```python
from build123d import *

# Parameters (mm, degrees)
ESBO_O1_R                = 1.5
ESBO_O1_W                = 5
ESBO_O1_H                = 35
RESSALTO_EXTRUS_O1_DEPTH = 3
ESBO_O2_W                = 25
ESBO_O2_H                = 5
RESSALTO_EXTRUS_O2_DEPTH = 15
FILETE5_R                = 5
FILETE6_R                = 5
FILETE7_R                = 5
FILETE8_R                = 5
ESBO_O3_R                = 1
ESBO_O3_W                = 4
ESBO_O3_H                = 4
CORTE_EXTRUS_O1_DEPTH    = 5
CORTE_EXTRUS_O2_START    = -5
ESBO_O4_R                = 1
ESBO_O4_W                = 4
ESBO_O4_H                = 4
CORTE_EXTRUS_O2_DEPTH    = 5


with BuildPart() as part:
    # Esboço1 → Ressalto-extrusão1 (new body)
    with BuildSketch(Plane.XY):
        Polygon((-24.430369357, 7.066666667), (10.569630643, 7.066666667), (10.569630643, 2.066666667), (5.569630643, 2.066666667), (5.569630643, -32.933333333), (10.569630643, -32.933333333), (10.569630643, -37.933333333), (-24.430369357, -37.933333333), (-24.430369357, -32.933333333), (-19.430369357, -32.933333333), (-19.430369357, 2.066666667), (-24.430369357, 2.066666667), align=None)
        with Locations((-14.430369357, -4.933333333)):
            Circle(ESBO_O1_R, mode=Mode.SUBTRACT)
        with Locations((-14.430369357, -11.933333333)):
            Circle(ESBO_O1_R, mode=Mode.SUBTRACT)
        with Locations((-14.430369357, -18.933333333)):
            Circle(ESBO_O1_R, mode=Mode.SUBTRACT)
        with Locations((0.569630643, -4.933333333)):
            Circle(ESBO_O1_R, mode=Mode.SUBTRACT)
        with Locations((0.569630643, -18.933333333)):
            Circle(ESBO_O1_R, mode=Mode.SUBTRACT)
        with Locations((0.569630643, -25.933333333)):
            Circle(ESBO_O1_R, mode=Mode.SUBTRACT)
        with Locations((-14.430369357, -25.933333333)):
            Circle(ESBO_O1_R, mode=Mode.SUBTRACT)
        with Locations((0.569630643, -11.933333333)):
            Circle(ESBO_O1_R, mode=Mode.SUBTRACT)
        with Locations((-21.930369357, 4.566666667)):
            Circle(ESBO_O1_R, mode=Mode.SUBTRACT)
        with Locations((8.069630643, 4.566666667)):
            Circle(ESBO_O1_R, mode=Mode.SUBTRACT)
        with Locations((-21.930369357, -35.433333333)):
            Circle(ESBO_O1_R, mode=Mode.SUBTRACT)
        with Locations((8.069630643, -35.433333333)):
            Circle(ESBO_O1_R, mode=Mode.SUBTRACT)
        with Locations((-6.930369357, -15.433333333)):
            Rectangle(ESBO_O1_W, ESBO_O1_H, mode=Mode.SUBTRACT)
    extrude(amount=-RESSALTO_EXTRUS_O1_DEPTH)

    # Esboço2 → Ressalto-extrusão2 (add)
    with BuildSketch(Plane.XY):
        with Locations((-6.930369357, 4.566666667)):
            Rectangle(ESBO_O2_W, ESBO_O2_H)
        with Locations((-6.930369357, -35.433333333)):
            Rectangle(ESBO_O2_W, ESBO_O2_H)
    extrude(amount=RESSALTO_EXTRUS_O2_DEPTH)

    # Filete5
    filete5_edges = [part.edges().sort_by_distance(p)[0] for p in [
        (5.569630643, -35.433333333, 15),
    ]]
    fillet(filete5_edges, radius=FILETE5_R)

    # Filete6
    filete6_edges = [part.edges().sort_by_distance(p)[0] for p in [
        (-19.430369357, -35.433333333, 15),
    ]]
    fillet(filete6_edges, radius=FILETE6_R)

    # Filete7
    filete7_edges = [part.edges().sort_by_distance(p)[0] for p in [
        (-19.430369357, 4.566666667, 15),
    ]]
    fillet(filete7_edges, radius=FILETE7_R)

    # Filete8
    filete8_edges = [part.edges().sort_by_distance(p)[0] for p in [
        (5.569630643, 4.566666667, 15),
    ]]
    fillet(filete8_edges, radius=FILETE8_R)

    # Esboço3 → Corte-extrusão1 (cut)
    with BuildSketch(Plane(origin=(0, -37.933333333, 0), x_dir=(-1, 0, 0), z_dir=(0, -1, 0))):
        with Locations(Location((13.180369357, -6, 0), (0, 0, 180))):
            Circle(ESBO_O3_R)
        with Locations(Location((0.680369357, -6.000000354, 0), (0, 0, 180))):
            Circle(ESBO_O3_R)
        with Locations((6.930369357, -6)):
            Rectangle(ESBO_O3_W, ESBO_O3_H)
    extrude(amount=-CORTE_EXTRUS_O1_DEPTH, mode=Mode.SUBTRACT)

    # Esboço4 → Corte-extrusão2 (cut)
    with BuildSketch(Plane(origin=(0, 7.066666667, 0), x_dir=(1, 0, 0), z_dir=(0, 1, 0)).offset(CORTE_EXTRUS_O2_START)):
        with Locations((-13.180369357, -6)):
            Circle(ESBO_O4_R)
        with Locations(Location((-0.680369357, -6, 0), (0, 0, 359.999979706))):
            Circle(ESBO_O4_R)
        with Locations((-6.930369357, -6)):
            Rectangle(ESBO_O4_W, ESBO_O4_H)
    extrude(amount=CORTE_EXTRUS_O2_DEPTH, mode=Mode.SUBTRACT)


solid = part.part
```
The listing builds one solid part. Answer for the finished solid, in the listing's coordinates (mm). A direction names the side the tool comes from. Give positions to 0.01 mm unless a question says otherwise; leave off trailing zeros. Loops run counter-clockwise (first coordinate to the right, second up) from the corner with the lowest first, then second, coordinate; pieces in that order, holes last. Notation, with made-up numbers: (-37, 6.5) - (-33, 6.5) arc R22 ccw to (-33, 28.5) - close; hole circle Ø2 at (60, 59). An arc over 180 degrees is marked (long way). Answer as CSV lines item,"result". Start each with the question number.
Item 1: For faces 1 (the face through (-23, 6, 0)), 2 (the face through (5.57, -35, 5)), 3 (the face through (8, 2.067, -1)), 4 (the face through (-4.93, 5, 6)), 5 (the face through (-19.43, -16, -1)), determine the directions among +Z, -Z, +X, -X, +Y, -Y from which every point of the face is accessible in a straight line to the end or side of a thin tool.
Item 2: A cutting plane is placed at C-C on z = 6. Count the separate pieces of the cut face and the enclosed holes in it, then the cut area to 3 significant figures.
Item 3: A cutting plane is placed at A-A on z = 3.25. Determine the outline of the cut face in (x, y), then the cut area to 3 significant figures.
Item 4: The mould has two halves that part along X. Classify faces 6 (the face through (-7, 7.067, 2)), 7 (the face through (-0.81, 4.53, 5.01)), 8 (the face through (-17.9, -35.4, 13.6)), 9 (the face through (10.57, 5, -1)): +X half, -X half, draft (parallel to the pull), parting line (faces both ways), or undercut.
Item 5: Find the intervals of material crossed by line 1 (X direction, y = -3, z = -0.5); line 2 (Y direction, x = -12.5, z = 9.5); line 3 (Y direction, x = -15, z = -0.25), in increasing order. Write a range as from..to.
Item 6: A cutting plane is placed at D-D on y = -28.5. Determine the outline of the cut face in (x, z).
Item 7: A cutting plane is placed at B-B on x = -8. Determine the outline of the cut face in (y, z), then the cut area to 3 significant figures.
Item 8: Each of these flat-tipped pins is pushed along its axis until it touches: pin 1 (4 mm diameter, centred on y = 4, z = 6.5, fed in from -X); pin 2 (12 mm diameter, centred on x = -17, y = -10.5, fed in from +Z); pin 3 (8 mm diameter, centred on y = -21, z = 0, fed in from +X). Where does it stop, or does it pass through?
Found:
1,face 1,"+Z, -X, +Y, -Y"
1,face 2,"+Z, +X, +Y, -Y"
1,face 3,"+Z, -Z, +X"
1,face 4,"+Y, -Y"
1,face 5,"+Z, -Z, -X"
2,separate pieces,"8"
2,enclosed holes,"0"
2,area,"170 mm^2"
3,outline,"(-19.43, -37.93) - (5.57, -37.93) - (5.57, -32.93) - (-19.43, -32.93) - close; (-19.43, 2.07) - (5.57, 2.07) - (5.57, 7.07) - (-19.43, 7.07) - close"
3,area,"250 mm^2"
4,face 6,"draft"
4,face 7,"undercut"
4,face 8,"-X half"
4,face 9,"+X half"
5,line 1,"x = -19.43..-9.43, -4.43..5.57"
5,line 2,"y = -37.93..-32.93, 2.07..7.07"
5,line 3,"y = -37.93..-27.32, -24.55..-20.32, -17.55..-13.32, -10.55..-6.32, -3.55..7.07"
6,outline,"(-19.43, -3) - (-9.43, -3) - (-9.43, 0) - (-19.43, 0) - close; (-4.43, -3) - (5.57, -3) - (5.57, 0) - (-4.43, 0) - close"
7,outline,"(-37.93, -3) - (-32.93, -3) - (-32.93, 4) - (-37.93, 4) - close; (-37.93, 8) - (-32.93, 8) - (-32.93, 15) - (-37.93, 15) - close; (2.07, -3) - (7.07, -3) - (7.07, 4) - (2.07, 4) - close; (2.07, 8) - (7.07, 8) - (7.07, 15) - (2.07, 15) - close"
7,area,"140 mm^2"
8,pin 1,"stops at x = -19.43"
8,pin 2,"stops at z = 0"
8,pin 3,"stops at x = 5.57"
